For this review, use the dimensioned drawing (mm, ordinates from the lowest corner) and the shaded views. Coordinates: 2 decimals unless noted, no trailing zeros. Write each loop counter-clockwise with the first axis right and the second up, starting at its lowest first coordinate (ties: lowest second). Pieces come first, ordered by that corner, then holes. Notation, with made-up numbers: (24.25, 40.5) -> (35.25, 40.5) arc R4 ccw to (35.25, 44.5) -> close; hole circle Ø5 at (-27, 16.5). An arc over 180 degrees is marked (long way). Put each result on its own line as item: value. Start each with the question number.
Item 1: To check wall thickness, follow L1, parallel to X at y = 2.85, z = 33.5; L2, parallel to X at y = 1.2, z = 40; L3, parallel to Z at x = 8, y = 3.4. State the ranges of each line that lie inside material, in increasing order.
Item 2: Consider section C-C on y = 1.25. Give the number of separate pieces and of enclosed holes in the cut face, and give its area (3 significant figures).
Item 3: Consider section B-B on x = 38.5. Give the boundary of the cut face in (y, z), and give its area (3 significant figures).
Item 4: Consider section A-A on z = 8. Give the boundary of the cut face in (x, y), and give its area (3 significant figures).
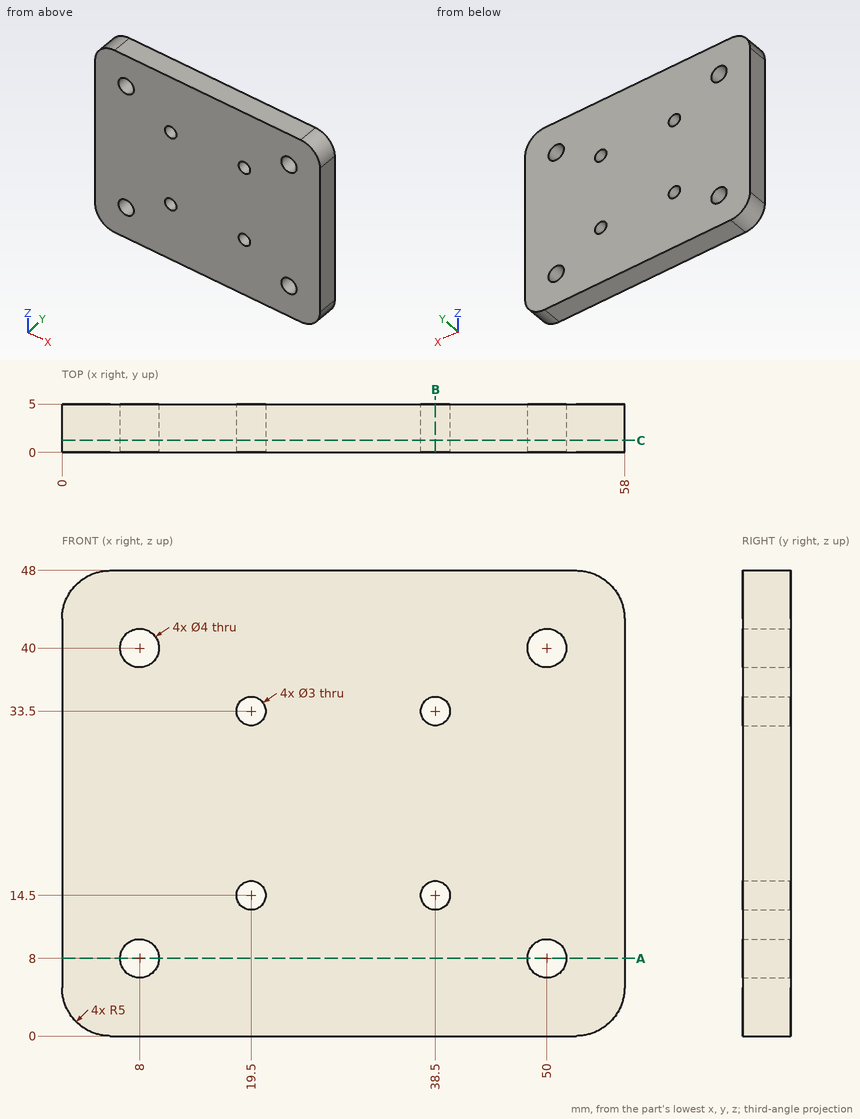
Return value:
1. L1: 0 to 18, 21 to 37, 40 to 58
1. L2: 0 to 6, 10 to 48, 52 to 58
1. L3: 0 to 6, 10 to 38, 42 to 48
2. separate pieces: 1
2. enclosed holes: 8
2. area: 2,680 mm^2
3. outline: (0, 0) -> (5, 0) -> (5, 13) -> (0, 13) -> close; (0, 16) -> (5, 16) -> (5, 32) -> (0, 32) -> close; (0, 35) -> (5, 35) -> (5, 48) -> (0, 48) -> close
3. area: 210 mm^2
4. outline: (0, 0) -> (6, 0) -> (6, 5) -> (0, 5) -> close; (10, 0) -> (48, 0) -> (48, 5) -> (10, 5) -> close; (52, 0) -> (58, 0) -> (58, 5) -> (52, 5) -> close
4. area: 250 mm^2
